```python
from build123d import *

# Parameters (mm, degrees)
BOSS_EXTRUDE1_DEPTH        = 3.175
F_6_CLEARANCE_HOLE1_D      = 4.3053
F_1_2_0_5_DIAMETER_HOLE1_D = 12.7


with BuildPart() as part:
    # Sketch1 → Boss-Extrude1 (new body)
    with BuildSketch(Plane.XY):
        with BuildLine():
            Line((0, 0), (0, 44.45))
            Line((0, 44.45), (-15.875, 44.45))
            ThreePointArc((-15.875, 44.45), (-18.12006403, 45.37993597), (-19.05, 47.625))
            Line((-19.05, 47.625), (-19.05, 118.745))
            ThreePointArc((-19.05, 118.745), (-18.12006403, 120.99006403), (-15.875, 121.92))
            Line((-15.875, 121.92), (0, 121.92))
            Line((0, 121.92), (0, 153.67))
            Line((0, 153.67), (-38.1, 153.67))
            Line((-38.1, 153.67), (-38.1, 0))
            Line((-38.1, 0), (0, 0))
        make_face()
    extrude(amount=BOSS_EXTRUDE1_DEPTH)

    # #6 Clearance Hole1 (through all)
    with Locations(Plane(origin=(0, 0, 0), x_dir=(-1, 0, 0), z_dir=(0, 0, -1))):
        with Locations((28.575, 9.525), (19.05, 146.05)):
            Hole(F_6_CLEARANCE_HOLE1_D / 2)

    # 1/2 (0.5) Diameter Hole1 (through all)
    with Locations(Plane(origin=(0, 0, 0), x_dir=(-1, 0, 0), z_dir=(0, 0, -1))):
        with Locations((13.97, 16.51)):
            Hole(F_1_2_0_5_DIAMETER_HOLE1_D / 2)


solid = part.part
```
CAD build for the part. Positions are in the model's coordinates, mm. A direction names the side the tool comes from. Round coordinates to 2 decimals unless told otherwise and drop trailing zeros. Write each loop counter-clockwise with the first axis right and the second up, starting at its lowest first coordinate (ties: lowest second). Pieces come first, ordered by that corner, then holes.
Item 1: Band-saw the part on C-C on x = -13.97. Write the cut outline in (y, z) (3 decimals).
Filled in:
outline: (0, 0) - (10.16, 0) - (10.16, 3.175) - (0, 3.175) - close; (22.86, 0) - (44.45, 0) - (44.45, 3.175) - (22.86, 3.175) - close; (121.92, 0) - (153.67, 0) - (153.67, 3.175) - (121.92, 3.175) - close
Item 2: Tool access for faces 1 (the flat face through (-19.05, 83, 2)), 2 (the flat face through (-19, 153.67, 2)): list every direction of +Z, -Z, +X, -X, +Y, -Y with a clear straight run to the whole face (end or side of a thin tool).
Filled in:
face 1: +Z, -Z, +X
face 2: +Z, -Z, +X, -X, +Y
Item 3: Drop a flat-ended pin along its axis: pin 1 Ø20.5 at (x, y) = (-13.97, 16.51) entering from +Z (3 decimals). Give the stop position or say it passes through.
Filled in:
pin 1: stops at z = 3.175
Item 4: Band-saw the part on A-A on x = -5. Write the cut outline in (y, z) (3 decimals), then the cut area to 3 significant figures.
Filled in:
outline: (0, 0) - (44.45, 0) - (44.45, 3.175) - (0, 3.175) - close; (121.92, 0) - (153.67, 0) - (153.67, 3.175) - (121.92, 3.175) - close
area: 242 mm2
Item 5: Band-saw the part on B-B on y = 146.05. Write the cut outline in (x, z) (3 decimals), then the cut area to 3 significant figures.
Filled in:
outline: (-38.1, 0) - (-21.203, 0) - (-21.203, 3.175) - (-38.1, 3.175) - close; (-16.897, 0) - (0, 0) - (0, 3.175) - (-16.897, 3.175) - close
area: 107 mm2
Item 6: Mould opens along X. For faces 3 (the cylindrical face through (-18.1, 45.36, 1.57)), 4 (the cylindrical face through (-14.797, 22.806, 1.61)), 5 (the cylindrical face through (-19.52, 143.95, 1.61)), 6 (the flat face through (-8, 121.92, 2)) say: released by +X, released by -X, zero draft, split by the parting line, or undercut.
Filled in:
face 3: released by +X
face 4: undercut
face 5: undercut
face 6: zero draft
Item 7: Drill centre lines: L1, parallel to Y at x = -13.97, z = 0.7; L2, parallel to Y at x = -2, z = 3.05; L3, parallel to X at y = 60, z = 2.4. Where is each one in solid material? Low to high.
Filled in:
L1: y = 0 to 10.16, 22.86 to 44.45, 121.92 to 153.67
L2: y = 0 to 44.45, 121.92 to 153.67
L3: x = -38.1 to -19.05
Item 8: Band-saw the part on D-D on z = 0.6. Write the cut outline in (x, y) (3 decimals).
Filled in:
outline: (-38.1, 0) - (0, 0) - (0, 44.45) - (-15.875, 44.45) arc R3.175 cw to (-19.05, 47.625) - (-19.05, 118.745) arc R3.175 cw to (-15.875, 121.92) - (0, 121.92) - (0, 153.67) - (-38.1, 153.67) - close; hole circle Ø4.305 at (-28.575, 9.525); hole circle Ø4.305 at (-19.05, 146.05); hole circle Ø12.7 at (-13.97, 16.51)
